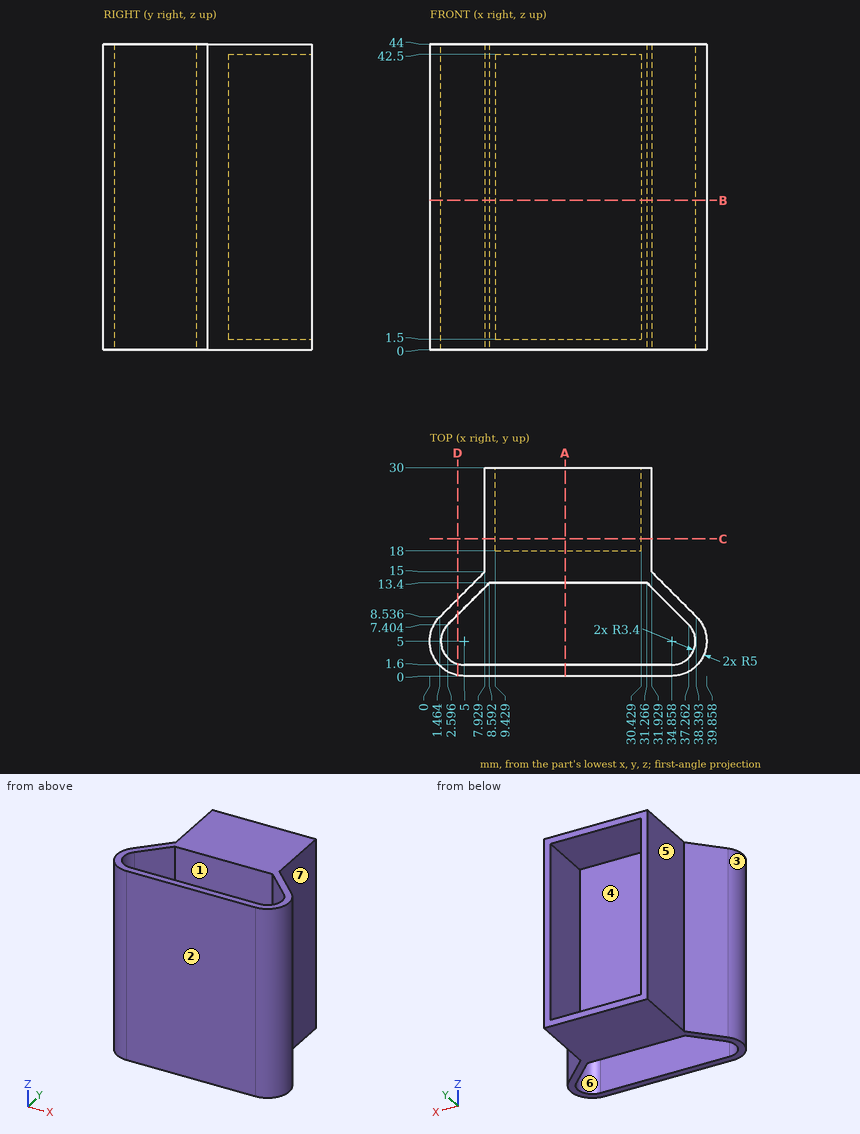
Check sheet for the drawn part. Datum: minimum x, y, z corner. Units: mm. A direction names the side the tool comes from. Coordinates: 2 decimals unless noted, no trailing zeros. Order: outer loops, then holes, each group sorted by start corner. A loop starts at its lowest first (then second) coordinate and runs counter-clockwise, first axis right, second up. Notation, with made-up numbers: (85, 6) - (144, 6) arc R20 cw to (144, 40) - close; hole circle Ø2 at (38, 38.25). An arc over 180 degrees is marked (long way). Return JSON: item names as keys, results as strings.
(1) Section check D-D, the plane x = 4. Record the cut outline in (y, z).
Filled sheet:
{"outline": "(0.1, 0) - (1.75, 0) - (1.75, 44) - (0.1, 44) - close; (8.81, 0) - (11.07, 0) - (11.07, 44) - (8.81, 44) - close"}
(2) Thickness scan on line 1 along X through (y, z) = (5.25, 25.5); line 2 along Y through (x, z) = (21.5, 20); line 3 along Y through (x, z) = (30.5, 17.5). Record the ranges inside material, lowest first.
Filled sheet:
{"line 1": "x = 0.01 to 1.61, 38.25 to 39.85", "line 2": "y = 0 to 1.6, 13.4 to 18", "line 3": "y = 0 to 1.6, 13.4 to 30"}
(3) Access from +Z, -Z, +X, -X, +Y, -Y to the whole of each face (thin tool, end or side, straight path). Record for the marked faces 4, 5, 6 and 7.
Filled sheet:
{"face 4": "+Y", "face 5": "+Z, -Z, -X, +Y", "face 6": "+Z, -Z", "face 7": "+Z, -Z, +X, +Y"}
(4) Section check C-C, the plane y = 19.75. Record the cut outline in (x, z), and give its area (3 significant figures).
Filled sheet:
{"outline": "(7.93, 0) - (31.93, 0) - (31.93, 44) - (7.93, 44) - close; hole (9.43, 1.5) - (30.43, 1.5) - (30.43, 42.5) - (9.43, 42.5) - close", "area": "195 mm^2"}
(5) Mould release check, pull along X, two halves, no side actions. Record for the marked faces 1, 2 and 3: pulls with the +X half, pulls with the -X half, needs draft (parallel to the pull), parting line crosses it, or undercut.
Filled sheet:
{"face 1": "undercut", "face 2": "needs draft", "face 3": "pulls with the -X half"}
(6) Section check A-A, the plane x = 19.5. Record the cut outline in (y, z), and give its area (3 significant figures).
Filled sheet:
{"outline": "(0, 0) - (1.6, 0) - (1.6, 44) - (0, 44) - close; (13.4, 0) - (30, 0) - (30, 1.5) - (18, 1.5) - (18, 42.5) - (30, 42.5) - (30, 44) - (13.4, 44) - close", "area": "309 mm^2"}
(7) Go/stop test with flat-tipped pins: pin 1 (1.5 mm diameter, centred on y = 16.5, z = 32.5, fed in from -X); pin 2 (10 mm diameter, centred on y = 16.5, z = 21.5, fed in from -X); pin 3 (9 mm diameter, centred on x = 23.5, z = 20.5, fed in from +Y). Record where each tip stops, or that it passes through.
Filled sheet:
{"pin 1": "stops at x = 7.93", "pin 2": "stops at x = 4.43", "pin 3": "stops at y = 18"}
(8) Section check B-B, the plane z = 21.5. Record the cut outline in (x, y) (1 decimal).
Filled sheet:
{"outline": "(1.5, 8.5) arc R5 ccw to (5, 0) - (34.9, 0) arc R5 ccw to (38.4, 8.5) - (31.9, 15) - (31.9, 30) - (30.4, 30) - (30.4, 18) - (9.4, 18) - (9.4, 30) - (7.9, 30) - (7.9, 15) - close; hole (2.6, 7.4) arc R3.4 ccw to (5, 1.6) - (34.9, 1.6) arc R3.4 ccw to (37.3, 7.4) - (31.3, 13.4) - (8.6, 13.4) - close"}
